The figure shows three views and two pictorial views of one solid part (mm, origin at its lowest corner). Answer the questions. A direction names the side the tool comes from. Round coordinates to 2 decimals unless told otherwise and drop trailing zeros. Loops run counter-clockwise (first coordinate to the right, second up) from the corner with the lowest first, then second, coordinate; pieces in that order, holes last. Notation, with made-up numbers: (-19, 69) -> (7, 69) arc R16 ccw to (7, 93) -> close; hole circle Ø10 at (6, 72.5). An arc over 180 degrees is marked (long way). Use a Markdown table: item, result. Add a question column.
Q1. For a pull along X with two mould halves and no side action, classify the marked faces 3, 4, 5 and 6 as released by +X, released by -X, zero draft, split by the parting line, or undercut.
Q2. Which of the six approach directions +Z, -Z, +X, -X, +Y, -Y give full straight-line access (tool end or side, diameter ignored) to the marked faces 1 and 2?
Q3. Section D-D on y = 4.5 is taken. Give the number of separate pieces and of enclosed holes in the cut face.
Q4. Section A-A on y = 19.05 is taken. Give the vertices of the cut face in (x, z), then the cut area to 3 significant figures.
Q5. Section B-B on x = 19.05 is taken. Give the vertices of the cut face in (y, z).
Q6. Consider line 1 (X direction, y = 4.5, z = 19.05); line 2 (Y direction, x = 5.75, z = 26.5). Determine where each line is inside the solid, lowest interval first.
Q7. Given pin 1 Ø1 at (x, y) = (18.5, 23.5) entering from -Z; pin 2 Ø2.5 at (x, z) = (19.05, 19.05) entering from +Y; pin 3 Ø10 at (x, y) = (12.5, 14) entering from +Z; pin 4 Ø5.5 at (x, z) = (6.35, 19.05) entering from +Y, each flat-ended and moving along its own axis, determine where each tip first touches the part or whether it passes through.
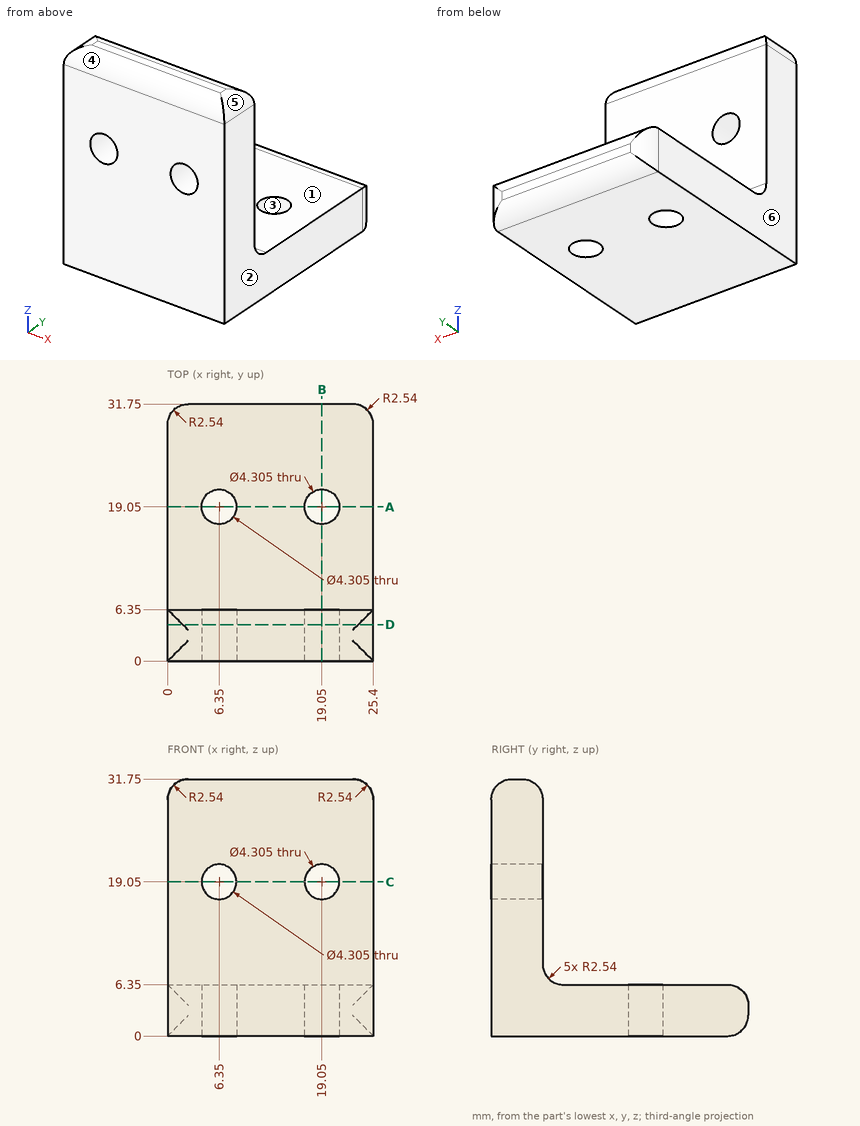
Checked values:
| question | item | result |
|---|---|---|
| 1 | face 3 | undercut |
| 1 | face 4 | zero draft |
| 1 | face 5 | released by +X |
| 1 | face 6 | released by -X |
| 2 | face 1 | +Z, +X, -X, +Y |
| 2 | face 2 | +Z, -Z, +X, +Y, -Y |
| 3 | separate pieces | 1 |
| 3 | enclosed holes | 2 |
| 4 | outline | (0, 0) -> (4.2, 0) -> (4.2, 6.35) -> (0, 6.35) -> close; (8.5, 0) -> (16.9, 0) -> (16.9, 6.35) -> (8.5, 6.35) -> close; (21.2, 0) -> (25.4, 0) -> (25.4, 6.35) -> (21.2, 6.35) -> close |
| 4 | area | 107 mm2 |
| 5 | outline | (0, 0) -> (16.9, 0) -> (16.9, 6.35) -> (8.89, 6.35) arc R2.54 cw to (6.35, 8.89) -> (6.35, 16.9) -> (0, 16.9) -> close; (0, 21.2) -> (6.35, 21.2) -> (6.35, 29.21) arc R2.54 ccw to (3.81, 31.75) -> (2.54, 31.75) arc R2.54 ccw to (0, 29.21) -> close; (21.2, 0) -> (29.21, 0) arc R2.54 ccw to (31.75, 2.54) -> (31.75, 3.81) arc R2.54 ccw to (29.21, 6.35) -> (21.2, 6.35) -> close |
| 6 | line 1 | x = 0 to 4.2, 8.5 to 16.9, 21.2 to 25.4 |
| 6 | line 2 | y = 0 to 6.35 |
| 7 | pin 1 | stops at z = 0 |
| 7 | pin 2 | passes through |
| 7 | pin 3 | stops at z = 6.35 |
| 7 | pin 4 | stops at y = 6.35 |
